Could you check a few things on this model? Use its own coordinates, in mm. Round coordinates to 2 decimals unless told otherwise and drop trailing zeros. Write each loop counter-clockwise with the first axis right and the second up, starting at its lowest first coordinate (ties: lowest second). Pieces come first, ordered by that corner, then holes. Notation, with made-up numbers: (-13.75, 28) -> (19.25, 28) arc R23 ccw to (19.25, 55) -> close; hole circle Ø2 at (42, 42.5). An arc over 180 degrees is marked (long way). Return JSON: item names as keys, results as strings.
Autodesk Fusion 360 part; units mm, degrees
sketch "Schizzo5" plane through (0, 0, 0) normal (0, 0, 1) x (1, 0, 0)
  line L0 (84.3315, 82.4519) -> (84.3315, -13.5481)
  circle A0 centre (89.3315, -11.0481) radius 1.5
  circle A1 centre (129.3315, 79.9519) radius 3
  line L1 (84.3315, 34.4519) -> (134.3315, 34.4519) construction
  circle A2 centre (109.3315, 79.9519) radius 1.5
  circle A3 centre (89.3315, 79.9519) radius 3
  circle A4 centre (89.3315, 79.9519) radius 1.5
  line L2 (134.3315, 82.4519) -> (84.3315, 82.4519)
  circle A5 centre (129.3315, 79.9519) radius 1.5
  circle A6 centre (109.3315, 79.9519) radius 3
  circle A7 centre (109.3315, 34.4519) radius 4.1
  circle A8 centre (109.3315, -11.0481) radius 1.5
  line L3 (134.3315, -13.5481) -> (134.3315, 82.4519)
  line L4 (89.3315, 82.4519) -> (89.3315, -13.5481) construction
  circle A9 centre (89.3315, -11.0481) radius 3
  circle A10 centre (109.3315, -11.0481) radius 3
  circle A11 centre (129.3315, -11.0481) radius 1.5
  line L5 (84.3315, -13.5481) -> (134.3315, -13.5481)
  circle A12 centre (129.3315, -11.0481) radius 3
  line L6 (84.3315, -11.0481) -> (134.3315, -11.0481) construction
  line L7 (109.3315, 82.4519) -> (109.3315, -13.5481) construction
  line L8 (109.3315, 34.4519) -> (109.3315, 59.4519) construction
  line L9 (113.8315, -0.5481) -> (104.8315, -0.5481)
  line L10 (104.8315, -0.5481) -> (104.8315, 19.4519)
  line L11 (104.8315, 19.4519) -> (113.8315, 19.4519)
  line L12 (113.8315, 19.4519) -> (113.8315, -0.5481)
  line L13 (113.8315, -0.5481) -> (104.8315, 19.4519) construction
  line L14 (104.8315, -0.5481) -> (113.8315, 19.4519) construction
  line L15 (113.8315, 49.4519) -> (113.8315, 69.4519)
  line L16 (104.8315, 49.4519) -> (113.8315, 49.4519)
  line L17 (104.8315, 69.4519) -> (104.8315, 49.4519)
  line L18 (113.8315, 69.4519) -> (104.8315, 69.4519)
  line L19 (104.8315, 69.4519) -> (113.8315, 49.4519) construction
  line L20 (113.8315, 69.4519) -> (104.8315, 49.4519) construction
  point P0 (127.8474, 12.2366)
  point P1 (109.3315, 9.4519)
  point P2 (109.3315, 59.4519)
  dimension "d221" = 50
  dimension "d222" = 96
  dimension "d223" = 2.5
  dimension "d224" = 20
  dimension "d225" = 3
  dimension "d226" = 6
  dimension "d227" = 3
  dimension "d228" = 6
  dimension "d229" = 8.2
  dimension "d354" = 9
  dimension "d355" = 20
  dimension "d356" = 50
extrude "Estrusione24" add sketch "Schizzo5" along normal blind 5 contours L0 A1 A3 L2 A6 L3 A9 A10 L5 A12 | A3 L2 | A9 L5 | L2 A6 | A10 L5 | A1 L2 | L5 A12 picked at (89.3689, 82.1172) picked at (89.3689, -13.2134) picked at (109.3689, 82.1172) picked at (109.3689, -13.2134) picked at (129.3689, 82.1172) picked at (129.3689, -13.2134)
extrude "Estrusione25" cut sketch "Schizzo5" against normal blind 3.2 from surface at 5 contours A3 L2 | A9 L5 | L2 A6 | A10 L5 | A1 L2 | L5 A12 picked at (89.3689, 82.1172) picked at (89.3689, -13.2134) picked at (109.3689, 82.1172) picked at (109.3689, -13.2134) picked at (129.3689, 82.1172) picked at (129.3689, -13.2134)
equation "d225 = d227"
equation "d226 = d228"
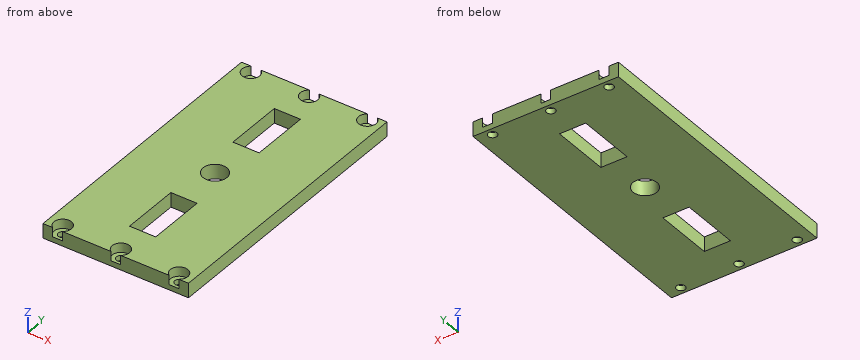
1) I want a section at C-C, the plane x = 129.5. Please give me the cut outline in (y, z).
Return value:
{"outline": "(-13.55, 0) -> (-12.54, 0) -> (-12.54, 1.8) -> (-13.55, 1.8) -> close; (-9.56, 0) -> (78.46, 0) -> (78.46, 1.8) -> (76.96, 1.8) -> (76.96, 5) -> (-8.05, 5) -> (-8.05, 1.8) -> (-9.56, 1.8) -> close; (81.44, 0) -> (82.45, 0) -> (82.45, 1.8) -> (81.44, 1.8) -> close"}
2) I want a section at A-A, the plane y = 68. Please give me the cut outline in (x, z), and give its area (3 significant figures).
Return value:
{"outline": "(84.33, 0) -> (104.83, 0) -> (104.83, 5) -> (84.33, 5) -> close; (113.83, 0) -> (134.33, 0) -> (134.33, 5) -> (113.83, 5) -> close", "area": "205 mm²"}
3) I want a section at B-B, the plane x = 109.5. Please give me the cut outline in (y, z), and give its area (3 significant figures).
Return value:
{"outline": "(-13.55, 0) -> (-12.54, 0) -> (-12.54, 1.8) -> (-13.55, 1.8) -> close; (-9.56, 0) -> (-0.55, 0) -> (-0.55, 5) -> (-8.05, 5) -> (-8.05, 1.8) -> (-9.56, 1.8) -> close; (19.45, 0) -> (30.36, 0) -> (30.36, 5) -> (19.45, 5) -> close; (38.55, 0) -> (49.45, 0) -> (49.45, 5) -> (38.55, 5) -> close; (69.45, 0) -> (78.46, 0) -> (78.46, 1.8) -> (76.96, 1.8) -> (76.96, 5) -> (69.45, 5) -> close; (81.44, 0) -> (82.45, 0) -> (82.45, 1.8) -> (81.44, 1.8) -> close", "area": "193 mm²"}
4) Will these pins go through, and if not, where does the flat tip stop? pin 1 Ø1.7 at (x, y) = (108, 78.5) entering from +Z; pin 2 Ø1.8 at (x, y) = (89.33, 79.95) entering from -Z.
Return value:
{"pin 1": "z = 1.8", "pin 2": "through"}
5) I want a section at D-D, the plane z = 3.9. Please give me the cut outline in (x, y).
Return value:
{"outline": "(84.33, -13.55) -> (87.67, -13.55) arc R3 cw (long way) to (90.99, -13.55) -> (107.67, -13.55) arc R3 cw (long way) to (110.99, -13.55) -> (127.67, -13.55) arc R3 cw (long way) to (130.99, -13.55) -> (134.33, -13.55) -> (134.33, 82.45) -> (130.99, 82.45) arc R3 cw (long way) to (127.67, 82.45) -> (110.99, 82.45) arc R3 cw (long way) to (107.67, 82.45) -> (90.99, 82.45) arc R3 cw (long way) to (87.67, 82.45) -> (84.33, 82.45) -> close; hole (104.83, -0.55) -> (113.83, -0.55) -> (113.83, 19.45) -> (104.83, 19.45) -> close; hole (104.83, 49.45) -> (113.83, 49.45) -> (113.83, 69.45) -> (104.83, 69.45) -> close; hole circle Ø8.2 at (109.33, 34.45)"}
6) If I drill on probe 1 along X at (y, z) = (3, 1.65); probe 2 along Y at (x, z) = (128.5, 0.8); probe 3 along Y at (x, z) = (107.5, 1.2), over which ranges is the centre line in solid material (lowest first)? Write a range as [from, to].
Return value:
{"probe 1": "[84.33, 104.83], [113.83, 134.33]", "probe 2": "[-13.55, -12.3], [-9.8, 78.7], [81.2, 82.45]", "probe 3": "[-13.55, -0.55], [19.45, 30.78], [38.12, 49.45], [69.45, 82.45]"}
